Here's how the part is built. I have some questions about the finished solid (model axes, mm). Coordinates: 2 decimals unless noted, no trailing zeros. Loops run counter-clockwise (first coordinate to the right, second up) from the corner with the lowest first, then second, coordinate; pieces in that order, holes last. Notation, with made-up numbers: M 21.25,22 L 58.25,22 A15 cw 58.25,34 Z; hole C -8.5,-31.5 d7. An arc over 180 degrees is marked long. Use CSV: the item, a comma, the result in double quotes. Start each with the question number.
Q1. Please list where these lines run through material, in increasing order: probe 1 along Y at (x, z) = (3, -3.45); probe 2 along Y at (x, z) = (23.5, -1.1). Write a range as [from, to].
Q2. If we section it at A-A (y = 9): Please give me the cut outline in (x, z).
Q3. If we section it at B-B (z = -1.9): Please give me the cut outline in (x, y).
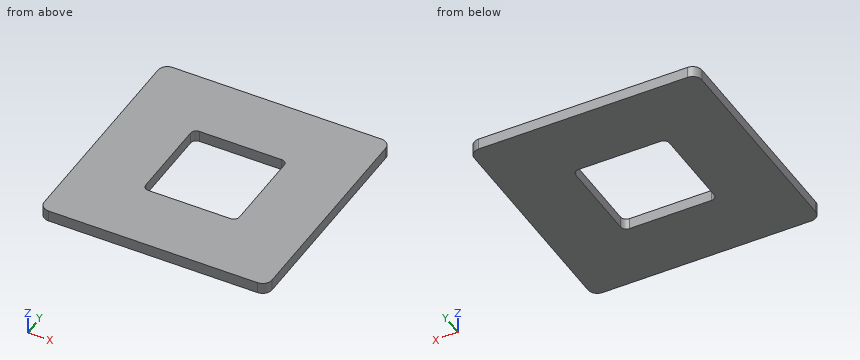
from build123d import *

# Parameters (mm, degrees)
F1_DEPTH = 6
F3_DEPTH = 10


with BuildPart() as f1:
    # F0 (on Top) → F1 (new body)
    with BuildSketch(Plane.XY):
        with BuildLine():
            Line((-55.8, -60.8), (55.8, -60.8))
            ThreePointArc((55.8, -60.8), (59.335534, -59.335534), (60.8, -55.8))
            Line((60.8, -55.8), (60.8, 55.8))
            ThreePointArc((60.8, 55.8), (59.335534, 59.335534), (55.8, 60.8))
            Line((55.8, 60.8), (-55.8, 60.8))
            ThreePointArc((-55.8, 60.8), (-59.335534, 59.335534), (-60.8, 55.8))
            Line((-60.8, 55.8), (-60.8, -55.8))
            ThreePointArc((-60.8, -55.8), (-59.335534, -59.335534), (-55.8, -60.8))
        make_face()
    extrude(amount=-F1_DEPTH)

    # F2 (on face) → F3 (cut)
    with BuildSketch(Plane.XY):
        with BuildLine():
            Line((-22, -25), (22, -25))
            ThreePointArc((22, -25), (24.12132, -24.12132), (25, -22))
            Line((25, -22), (25, 22))
            ThreePointArc((25, 22), (24.12132, 24.12132), (22, 25))
            Line((22, 25), (-22, 25))
            ThreePointArc((-22, 25), (-24.12132, 24.12132), (-25, 22))
            Line((-25, 22), (-25, -22))
            ThreePointArc((-25, -22), (-24.12132, -24.12132), (-22, -25))
        make_face()
    extrude(amount=-F3_DEPTH, mode=Mode.SUBTRACT)


solid = f1.part
Results below:
1,probe 1,"[-60.8, -25], [25, 60.8]"
1,probe 2,"[-60.8, -24.6], [24.6, 60.8]"
2,outline,"M -60.8,-6 L -25,-6 L -25,0 L -60.8,0 Z; M 25,-6 L 60.8,-6 L 60.8,0 L 25,0 Z"
3,outline,"M -60.8,-55.8 A5 ccw -55.8,-60.8 L 55.8,-60.8 A5 ccw 60.8,-55.8 L 60.8,55.8 A5 ccw 55.8,60.8 L -55.8,60.8 A5 ccw -60.8,55.8 Z; hole M -25,-22 A3 ccw -22,-25 L 22,-25 A3 ccw 25,-22 L 25,22 A3 ccw 22,25 L -22,25 A3 ccw -25,22 Z"
